The listing builds one solid part. Answer for the finished solid, in the listing's coordinates (mm). A direction names the side the tool comes from. Give positions to 0.01 mm unless a question says otherwise; leave off trailing zeros. Loops run counter-clockwise (first coordinate to the right, second up) from the corner with the lowest first, then second, coordinate; pieces in that order, holes last. Notation, with made-up numbers: (-29, -1.5) - (22, -1.5) arc R20 ccw to (22, 9.5) - close; hole circle Ø8 at (-1, 72.5). An arc over 180 degrees is marked (long way). Write each question's results on one line, items separated by ' | '.
from build123d import *

# Parameters (mm, degrees)
AUFSATZ_LINEAR_AUSTRAGEN1_DEPTH = 10
SKIZZE2_R                       = 1.75
SCHNITT_LINEAR_AUSTRAGEN1_DEPTH = 38
SKIZZE4_R                       = 2.2
SCHNITT_LINEAR_AUSTRAGEN3_DEPTH = 52.2
VERRUNDUNG1_R                   = 10
SKIZZE5_W                       = 5.5
SKIZZE5_H                       = 5.5
SCHNITT_LINEAR_AUSTRAGEN4_DEPTH = 2
FASE1_SIZE                      = 1.5
SCHNITT_LINEAR_AUSTRAGEN5_DEPTH = 11


with BuildPart() as part:
    # Skizze1 → Aufsatz-Linear austragen1 (new body)
    with BuildSketch(Plane.XY):
        with BuildLine():
            Line((0.5, -28.495613698), (0.5, -32.496153619))
            Line((0.5, -32.496153619), (0.5, -39.496153619))
            Line((0.5, -39.496153619), (4.5, -39.496153619))
            Line((4.5, -39.496153619), (4.5, -32.186953879))
            ThreePointArc((4.5, -32.186953879), (31.590882714, -7.633225356), (18.7, 26.581196361))
            Line((18.7, 26.581196361), (18.7, 51.5))
            Line((18.7, 51.5), (10.2, 51.5))
            Line((10.2, 51.5), (10.2, 31.5))
            Line((10.2, 31.5), (-10.2, 31.5))
            Line((-10.2, 31.5), (-10.2, 51.5))
            Line((-10.2, 51.5), (-18.7, 51.5))
            Line((-18.7, 51.5), (-18.7, 26.581196361))
            ThreePointArc((-18.7, 26.581196361), (-31.590882714, -7.633225356), (-4.5, -32.186953879))
            Line((-4.5, -32.186953879), (-4.5, -39.496153619))
            Line((-4.5, -39.496153619), (-0.5, -39.496153619))
            Line((-0.5, -39.496153619), (-0.5, -32.496153619))
            Line((-0.5, -32.496153619), (-0.5, -28.495613698))
            ThreePointArc((-0.5, -28.495613698), (0, 28.5), (0.5, -28.495613698))
        make_face()
    extrude(amount=AUFSATZ_LINEAR_AUSTRAGEN1_DEPTH)

    # Skizze2 → Schnitt-Linear austragen1 (cut, through all)
    with BuildSketch(Plane.ZY.offset(4.5)):
        with Locations((5, -35.841553749)):
            Circle(SKIZZE2_R)
    extrude(amount=-SCHNITT_LINEAR_AUSTRAGEN1_DEPTH, mode=Mode.SUBTRACT)

    # Skizze4 → Schnitt-Linear austragen3 (cut, through all)
    with BuildSketch(Plane.ZY.offset(18.7)):
        with Locations((5, 41.5)):
            Circle(SKIZZE4_R)
    extrude(amount=-SCHNITT_LINEAR_AUSTRAGEN3_DEPTH, mode=Mode.SUBTRACT)

    # Verrundung1
    verrundung1_edges = [part.edges().sort_by_distance(p)[0] for p in [
        (-18.7, 26.581196361, 5),
        (18.7, 26.581196361, 5),
    ]]
    fillet(verrundung1_edges, radius=VERRUNDUNG1_R)

    # Skizze5 → Schnitt-Linear austragen4 (cut)
    with BuildSketch(Plane.ZY.offset(4.5)):
        with Locations((5, -35.841553749)):
            Rectangle(SKIZZE5_W, SKIZZE5_H)
    extrude(amount=-SCHNITT_LINEAR_AUSTRAGEN4_DEPTH, mode=Mode.SUBTRACT)

    # Fase1
    fase1_edges = [part.edges().sort_by_distance(p)[0] for p in [
        (-18.7, 41.422906559, 0),
        (31.036620275, -9.642520517, 0),
        (-18.7, 41.422906559, 10),
        (18.7, 41.422906559, 0),
        (18.7, 41.422906559, 10),
        (31.036620275, -9.642520517, 10),
        (-31.036620275, -9.642520517, 0),
        (-31.036620275, -9.642520517, 10),
        (19.547693958, 27.316508696, 0),
        (19.547693958, 27.316508696, 10),
        (-19.547693958, 27.316508696, 0),
        (-19.547693958, 27.316508696, 10),
    ]]
    chamfer(fase1_edges, length=FASE1_SIZE)

    # Skizze6 → Schnitt-Linear austragen5 (cut, through all)
    with BuildSketch(Plane.XY):
        Polygon((0, -80.065943577), (0, 27.478555263), (-0.15, 27.478555263), (-0.15, 32.428870792), (0, 32.428870792), (0, 80.065943577), (51.694887104, 80.065943577), (51.694887104, -72.979708266), align=None)
    extrude(amount=SCHNITT_LINEAR_AUSTRAGEN5_DEPTH, mode=Mode.SUBTRACT)


solid = part.part
Item 1: A cutting plane is placed at C-C, the plane y = 0. Determine the outline of the cut face in (x, z).
Values found:
outline: (-32.5, 1.5) - (-31, 0) - (-28.5, 0) - (-28.5, 10) - (-31, 10) - (-32.5, 8.5) - close
Item 2: A cutting plane is placed at A-A, the plane y = 41.5. Determine the outline of the cut face in (x, z), plus the area to 4 significant figures.
Values found:
outline: (-18.7, 1.5) - (-17.2, 0) - (-10.2, 0) - (-10.2, 2.8) - (-18.7, 2.8) - close; (-18.7, 7.2) - (-10.2, 7.2) - (-10.2, 10) - (-17.2, 10) - (-18.7, 8.5) - close | area: 45.35 mm²
Item 3: For faces 1 (the face through (-4, -33.092, 5)), 2 (the face through (-28.496, -0.447, 4.93)), 3 (the face through (-18.7, 44, 5)), 4 (the face through (-5, 31.5, 5)), 5 (the face through (-23, 20, 0)), determine the directions among +Z, -Z, +X, -X, +Y, -Y from which every point of the face is accessible in a straight line to the end or side of a thin tool.
Values found:
face 1: -X | face 2: +Z, -Z, +X | face 3: +Z, -Z, -X, +Y | face 4: +Z, -Z, +X, +Y | face 5: -Z, +X, -X, +Y, -Y
Item 4: Flat-ended cylindrical pins translate along their axes: P1, Ø3.5, axis at y = 41.5, z = 5, coming from the +X side; P2, Ø6, axis at x = -16.5, z = 6, coming from the -Y side; P3, Ø1, axis at x = -3, z = 5, coming from the +Y side; P4, Ø5.5, axis at y = 45, z = 3.5, coming from the -X side. Find the tip coordinate at first contact, or state that the pin passes through.
Values found:
P1: passes through | P2: stops at y = -29.56 | P3: stops at y = 31.5 | P4: stops at x = -18.7
Item 5: Find the intervals of material crossed by line 1 along Y through (x, z) = (-1.2, 5); line 2 along Y through (x, z) = (-12.5, 5); line 3 along X through (y, z) = (-1, 2), in increasing order. Write a range as [from, to].
Values found:
line 1: y = [-39.5, -37.59], [-34.09, -28.47], [28.47, 31.5] | line 2: y = [-30, -25.61], [25.61, 39.3], [43.7, 51.5] | line 3: x = [-32.48, -28.48]
Item 6: For a pull along Y with two mould halves and no side action, classify faces 6 (the face through (-14, 51.5, 5)), 7 (the face through (-3, -39.496, 5)), 8 (the face through (-14.51, 39.352, 4.523)), 9 (the face through (-18, 41.6, 0.8)) as released by +Y, released by -Y, zero draft, split by the parting line, or undercut.
Values found:
face 6: released by +Y | face 7: released by -Y | face 8: undercut | face 9: zero draft
